Part model, mm, in its own coordinate system. A direction names the side the tool comes from. Coordinates: 2 decimals unless noted, no trailing zeros. Write each loop counter-clockwise with the first axis right and the second up, starting at its lowest first coordinate (ties: lowest second). Pieces come first, ordered by that corner, then holes. Notation, with made-up numbers: (60.25, 37) -> (65.25, 37) arc R23 cw to (65.25, 75) -> close; hole circle Ø11 at (46.5, 39). An arc over 180 degrees is marked (long way). Write item = value, one per line.
from build123d import *

# Parameters (mm, degrees)
F0_W     = 29.6439956874
F0_H     = 67.9221600294
F1_DEPTH = 23.876
F2_W     = 29.6439956874
F2_H     = 5.4683089256
F3_DEPTH = 40.64
F4_DEPTH = 28.956
F5_W     = 6.9073364139
F5_H     = 2.8780577704
F6_DEPTH = 3.302


with BuildPart() as f1:
    # F0 (on Front) → F1 (new body)
    with BuildSketch(Plane.XZ):
        with Locations((14.8219978437, 33.9610800147)):
            Rectangle(F0_W, F0_H)
    extrude(amount=F1_DEPTH)

    # F2 (on Front) → F3 (join)
    with BuildSketch(Plane.XZ):
        with Locations((14.8219978437, 53.6757744849)):
            Rectangle(F2_W, F2_H)
    extrude(amount=F3_DEPTH)

    # F4 (cut): a face of the model
    f4_faces = [f1.faces().sort_by_distance(p)[0] for p in [
        (14.8219978437, -40.64, 53.6757744849),
    ]]
    extrude(f4_faces, amount=-F4_DEPTH, mode=Mode.SUBTRACT)

    # F5 (on Top) → F6 (join)
    with BuildSketch(Plane.XY):
        with Locations((14.3902879208, 1.4390288852)):
            Rectangle(F5_W, F5_H)
    extrude(amount=F6_DEPTH)


solid = f1.part
Q1. Saw through at A-A on y = -16.25. Give the cut face in (x, z).
Model answer:
outline = (0, 0) -> (29.64, 0) -> (29.64, 50.94) -> (0, 50.94) -> close; (0, 56.41) -> (29.64, 56.41) -> (29.64, 67.92) -> (0, 67.92) -> close
Q2. Mould opens along Z. For faces 5 (the face through (15, -18, 56.41)), 6 (the face through (15, -10, 0)), 7 (the face through (10.937, 1, 2)) say: released by +Z, released by -Z, zero draft, split by the parting line, or undercut.
Model answer:
face_5 = undercut
face_6 = released by -Z
face_7 = zero draft
Q3. Saw through at C-C on z = 54. Give the cut face in (x, y), and give its area (3 significant figures).
Model answer:
outline = (0, -11.68) -> (29.64, -11.68) -> (29.64, 0) -> (0, 0) -> close
area = 346 mm²
Q4. Saw through at B-B on x = 25. Give the cut face in (y, z).
Model answer:
outline = (-23.88, 0) -> (0, 0) -> (0, 67.92) -> (-23.88, 67.92) -> (-23.88, 56.41) -> (-11.68, 56.41) -> (-11.68, 50.94) -> (-23.88, 50.94) -> close
Q5. Saw through at D-D on x = 14.5. Give the cut face in (y, z), and give its area (3 significant figures).
Model answer:
outline = (-23.88, 0) -> (2.88, 0) -> (2.88, 3.3) -> (0, 3.3) -> (0, 67.92) -> (-23.88, 67.92) -> (-23.88, 56.41) -> (-11.68, 56.41) -> (-11.68, 50.94) -> (-23.88, 50.94) -> close
area = 1,560 mm²
Q6. Pin check, flat tips, straight feed: pin 1 (3 mm diameter, centred on x = 19.5, z = 8, fed in from +Y); pin 2 (2.5 mm diameter, centred on x = 14.5, z = 54.5, fed in from -Y); pin 3 (0.9 mm diameter, centred on y = 1, z = 1.5, fed in from -X). Stop position of each tip, or through.
Model answer:
pin_1 = 0
pin_2 = -11.68
pin_3 = 10.94
Q7. Which spindle directions (+Z, -Z, +X, -X, +Y, -Y) get a long thin tool onto all of the face, cutting with end or side? Do faces 1 (the face through (15, -18, 50.942)), 2 (the face through (14, 1, 3.302)), 3 (the face through (17.844, 1, 2)), 4 (the face through (0, -12, 33)). Say none if no direction does.
Model answer:
face_1 = +X, -X, -Y
face_2 = +Z, +X, -X, +Y
face_3 = +Z, -Z, +X, +Y
face_4 = +Z, -Z, -X, +Y, -Y
Q8. Probe line 1 (Z direction, x = 18.5, y = -18.25); line 2 (Y direction, x = 2.5, z = 17); line 3 (Y direction, x = 7.5, z = 54). List the from-to ranges inside material, lowest first. Write a range as from..to.
Model answer:
line_1 = 0..50.94, 56.41..67.92
line_2 = -23.88..0
line_3 = -11.68..0
